Part model, mm, in its own coordinate system. A direction names the side the tool comes from. Coordinates: 2 decimals unless noted, no trailing zeros.
from build123d import *

# Parameters (mm, degrees)
SKETCH2_R           = 10
EXTRUDE1_DEPTH      = 2
EXTRUDE1_TAPER      = 41
SKETCH3_R           = 5.5
EXTRUDE2_DEPTH      = 4
EXTRUDE2_TAPER      = 15
SKETCH4_R           = 2.5
EXTRUDE3_DEPTH      = 1
SKETCH5_R           = 1.5
EXTRUDE4_DEPTH      = 24
EXTRUDE4_DEPTH_BACK = 15
SKETCH6_RX          = 6
SKETCH6_RY          = 4
EXTRUDE5_DEPTH      = 15
CIRPATTERN2_COUNT   = 8
SKETCH7_R           = 2.75
EXTRUDE6_DEPTH      = 7


with BuildPart() as part:
    # Sketch1 → Revolve1 (revolve)
    with BuildSketch(Plane(origin=(0, 0, 0), x_dir=(0, 0, -1), z_dir=(1, 0, 0))):
        Polygon((-3.75, 28.5), (-1.5, 28.5), (-1.5, 0), (1.5, 0), (1.5, 28.5), (3.75, 28.5), (3.75, 30.5), (2.75, 30.5), (2.75, 32.5), (-2.75, 32.5), (-2.75, 30.5), (-3.75, 30.5), align=None)
    revolve(axis=Axis((0, 0, 21.188406287), (0, 0, -1)))

    # Sketch2 → Extrude1 (add)
    with BuildSketch(Plane.XY.offset(1.5)):
        Circle(SKETCH2_R)
    extrude(amount=EXTRUDE1_DEPTH, taper=EXTRUDE1_TAPER)

    # Sketch3 → Extrude2 (add)
    with BuildSketch(Plane(origin=(0, 0, -1.5), x_dir=(-1, 0, 0), z_dir=(0, 0, -1))):
        Circle(SKETCH3_R)
    extrude(amount=EXTRUDE2_DEPTH, taper=EXTRUDE2_TAPER)

    # Sketch4 → Extrude3 (cut)
    with BuildSketch(Plane.XY.offset(3.5)):
        Circle(SKETCH4_R)
    extrude(amount=-EXTRUDE3_DEPTH, mode=Mode.SUBTRACT)

    # Sketch5 → Extrude4 (cut, two sides)
    with BuildSketch(Plane.XY.offset(2.5)) as extrude4_sk:
        Circle(SKETCH5_R)
    extrude(amount=EXTRUDE4_DEPTH, mode=Mode.SUBTRACT)
    extrude(extrude4_sk.sketch, amount=-EXTRUDE4_DEPTH_BACK, mode=Mode.SUBTRACT)

    # Sketch6 → Extrude5 (cut)
    with BuildSketch(Plane.XY.offset(1.5)):
        with Locations(Location((0, 21), (0, 0, 90))):
            Ellipse(SKETCH6_RX, SKETCH6_RY)
    extrude5 = extrude(amount=-EXTRUDE5_DEPTH, mode=Mode.SUBTRACT)

    # CirPattern2: Extrude5 ×8 about axis
    cirpattern2_axis = Axis((0, 0, 21.188406287), (0, 0, 1))
    for i in range(1, CIRPATTERN2_COUNT):
        add(extrude5.rotate(cirpattern2_axis, i * 360 / CIRPATTERN2_COUNT), mode=Mode.SUBTRACT)

    # Sketch7 → Extrude6 (cut)
    with BuildSketch(Plane(origin=(0, 0, -5.5), x_dir=(-1, 0, 0), z_dir=(0, 0, -1))):
        Circle(SKETCH7_R)
    extrude(amount=-EXTRUDE6_DEPTH, mode=Mode.SUBTRACT)


solid = part.part
Q1. Wall check: line 1 along Y through (x, z) = (11.5, -0.25); line 2 along Z through (x, y) = (-22, -12); line 3 along Y through (x, z) = (1, 1.25). Give the ranges that are in metal, low to high.
Results list:
line 1: y = -30.4 to -17.11, -10.01 to 10.01, 17.11 to 30.4
line 2: z = -1.5 to 1.5
line 3: y = -32.48 to -26.81, -15.19 to -2.56, 2.56 to 15.19, 26.81 to 32.48
Q2. Pin check, flat tips, straight feed: pin 1 Ø5 at (x, z) = (23.5, -2) entering from -Y; pin 2 Ø13 at (x, y) = (-2, -1.5) entering from +Z; pin 3 Ø4.5 at (x, y) = (-1, -0.5) entering from -Z; pin 4 Ø4 at (x, y) = (0, 0) entering from -Z. Stop position of each tip, or through.
Results list:
pin 1: stops at y = -24.8
pin 2: stops at z = 3.5
pin 3: stops at z = -5.5
pin 4: stops at z = 1.5
Q3. Which spindle directions (+Z, -Z, +X, -X, +Y, -Y) get a long thin tool onto all of the face, cutting with end or side? Do faces 1 (the face through (29, -10, 2.75)), 2 (the face through (-18.559, -24.204, -3.243)), 3 (the face through (-1.5, 0.07, 2.01)). Say none if no direction does.
Results list:
face 1: +Z
face 2: -Z
face 3: +Z, -Z
Q4. Mould opens along X. For faces 4 (the face through (0, -3, -5.5)), 5 (the face through (0, -2, 2.5)), 6 (the face through (9.76, 31, 0.04)), 7 (the face through (-6, 0, -1.5)) say: pulls with the +X half, pulls with the -X half, needs draft (parallel to the pull), parting line crosses it, or undercut.
Results list:
face 4: needs draft
face 5: undercut
face 6: parting line crosses it
face 7: undercut
Q5. Cut at A-A on y = 0. Count the separate pieces of the cut face and the enclosed holes in it, and give its area (3 significant figures).
Results list:
separate pieces: 4
enclosed holes: 0
area: 181 mm2
